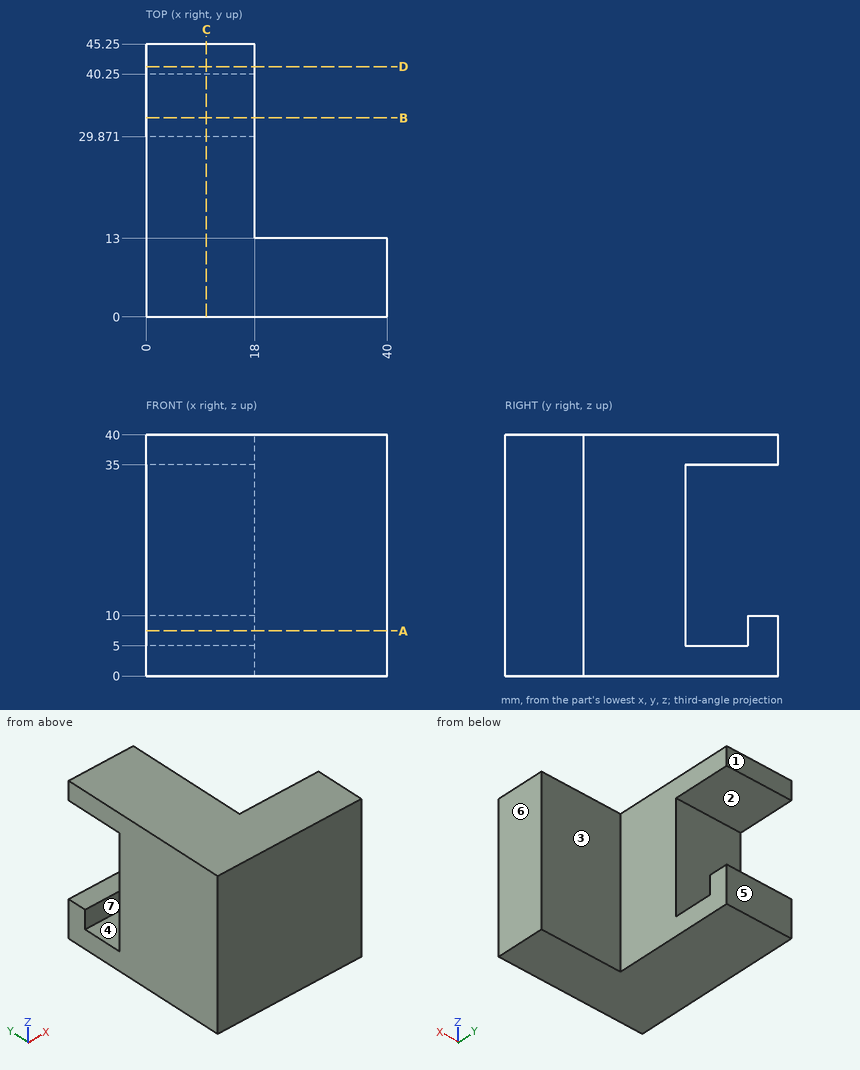
Print and shaded views of the part. All mm, measured from the part's lowest x, y and z. A direction names the side the tool comes from. Round coordinates to 2 decimals unless told otherwise and drop trailing zeros. Order: outer loops, then holes, each group sorted by start corner. A loop starts at its lowest first (then second) coordinate and runs counter-clockwise, first axis right, second up.
Q1. Two-plate mould, pull along Y, no slides. Class the marked faces 4, 5, 6 and 7: pulls with the +Y half, pulls with the -Y half, needs draft (parallel to the pull), parting line crosses it, or undercut.
Q2. Slice it at C-C (x = 10). Write the cut outline in (y, z).
Q3. Which spindle directions (+Z, -Z, +X, -X, +Y, -Y) get a long thin tool onto all of the face, cutting with end or side? Do the marked faces 1, 2 and 3. Say none if no direction does.
Q4. Drop flat-ended pins along their axis: pin 1 (6.5 mm diameter, centred on x = 32.5, z = 22.5, fed in from +Y); pin 2 (1.5 mm diameter, centred on y = 27, z = 25.5, fed in from +X). Give the stop position or say it passes through.
Q5. Slice it at A-A (z = 7.5). Write the cut outline in (x, y).
Q6. Slice it at D-D (y = 41.5). Write the cut outline in (x, z), and give its area (3 significant figures).
Q7. Slice it at B-B (y = 33). Write the cut outline in (x, z), and give its area (3 significant figures).
Q8. Wall check: L1, parallel to Y at x = 2, z = 15.5; L2, parallel to Z at x = 12, y = 31; L3, parallel to X at y = 19, z = 16.5. Give the ranges that are in metal, low to high.
Results below:
1. face 4: undercut
1. face 5: pulls with the +Y half
1. face 6: needs draft
1. face 7: undercut
2. outline: (0, 0) - (45.25, 0) - (45.25, 10) - (40.25, 10) - (40.25, 5) - (29.87, 5) - (29.87, 35) - (45.25, 35) - (45.25, 40) - (0, 40) - close
3. face 1: +Z, -Z, +X, -X, +Y
3. face 2: +X, -X, +Y
3. face 3: +Z, -Z, +X, +Y
4. pin 1: stops at y = 13
4. pin 2: stops at x = 18
5. outline: (0, 0) - (40, 0) - (40, 13) - (18, 13) - (18, 29.87) - (0, 29.87) - close; (0, 40.25) - (18, 40.25) - (18, 45.25) - (0, 45.25) - close
6. outline: (0, 0) - (18, 0) - (18, 10) - (0, 10) - close; (0, 35) - (18, 35) - (18, 40) - (0, 40) - close
6. area: 270 mm2
7. outline: (0, 0) - (18, 0) - (18, 5) - (0, 5) - close; (0, 35) - (18, 35) - (18, 40) - (0, 40) - close
7. area: 180 mm2
8. L1: y = 0 to 29.87
8. L2: z = 0 to 5, 35 to 40
8. L3: x = 0 to 18
